Can you work these out from the model? Positions are in its coordinate system, mm. A direction names the side the tool comes from. Round coordinates to 2 decimals unless told otherwise and drop trailing zeros. Order: outer loops, then holes, each group sorted by start corner. A loop starts at its lowest first (then second) coordinate and runs counter-clockwise, first axis right, second up. Notation, with made-up numbers: (-33, 60.5) -> (-16, 60.5) arc R32 cw to (-16, 87.5) -> close; hole circle Ø7 at (-1, 1). An arc over 180 degrees is marked (long way). One line per item, written item: value.
```python
from build123d import *

# Parameters (mm, degrees)
EXTRUDE_1_DEPTH     = 68
SKETCH_2_R          = 1.5
CUT_EXTRUDE_1_DEPTH = 60
SKETCH_3_W          = 30
SKETCH_3_H          = 4
EXTRUDE_2_DEPTH     = 40
EXTRUDE_3_DEPTH     = 30
CUT_EXTRUDE_2_DEPTH = 4
EXTRUDE_4_DEPTH     = 23
EXTRUDE_START       = -53
EXTRUDE_5_DEPTH     = 23
EXTRUDE_6_DEPTH     = 3
EXTRUDE_7_DEPTH     = 0.66666
SKETCH_17_W         = 17.087989765
SKETCH_17_H         = 19.996406133
EXTRUDE_9_DEPTH     = 12
SKETCH_19_R         = 1.8
CUT_EXTRUDE_3_DEPTH = 20
SKETCH_20_W         = 61.603006609
SKETCH_20_H         = 84.586869481
CUT_EXTRUDE_4_DEPTH = 65
SKETCH_21_W         = 7.494214953
SKETCH_21_H         = 26.873102225
CUT_EXTRUDE_5_DEPTH = 2
SKETCH_22_W         = 9.970658679
SKETCH_22_H         = 25.794738871
CUT_EXTRUDE_6_DEPTH = 2
EXTRUDE_10_DEPTH    = 4
FILLET_1_R          = 1
FILLET_2_R          = 1


with BuildPart() as part:
    # 草图1 → 凸台-拉伸1 (new body)
    with BuildSketch(Plane(origin=(0, 0, 0), x_dir=(0, 0, -1), z_dir=(1, 0, 0))):
        Polygon((0, 0), (0, 4), (-10, 4), (-10, 7), (0, 7), (0, 10), (-14, 10), (-14, 0), align=None)
    extrude(amount=EXTRUDE_1_DEPTH)

    # 草图2 → 切除-拉伸1 (cut)
    with BuildSketch(Plane(origin=(0, 10, 0), x_dir=(1, 0, 0), z_dir=(0, 1, 0))):
        with Locations(Location((5, -3.5, 0), (0, 0, 270))):
            Circle(SKETCH_2_R)
        with Locations(Location((63, -3.5, 0), (0, 0, 270))):
            Circle(SKETCH_2_R)
    extrude(amount=-CUT_EXTRUDE_1_DEPTH, mode=Mode.SUBTRACT)

    # 草图3 → 凸台-拉伸2 (add)
    with BuildSketch(Plane.XZ):
        with Locations((34, 12)):
            Rectangle(SKETCH_3_W, SKETCH_3_H)
    extrude(amount=-EXTRUDE_2_DEPTH)

    # 草图4 → 凸台-拉伸3 (add)
    with BuildSketch(Plane(origin=(49, 0, 0), x_dir=(0, 0, -1), z_dir=(1, 0, 0))):
        Polygon((-14, 40), (-26.357684131, 54.727314459), (-23.293506358, 57.298464898), (-10, 41.455880937), (-10, 40), align=None)
    extrude(amount=-EXTRUDE_3_DEPTH)

    # 草图5 → 切除-拉伸2 (cut)
    with BuildSketch(Plane(origin=(0, 9.633382176, -11.480617817), x_dir=(1, 0, 0), z_dir=(0, -0.6427876096865429, 0.7660444431189751))):
        with BuildLine():
            Line((25.25, 55.318123989), (25.25, 43.864814933))
            ThreePointArc((25.25, 43.864814933), (23.75, 42.364814933), (22.25, 43.864814933))
            Line((22.25, 43.864814933), (22.25, 55.318123989))
            ThreePointArc((22.25, 55.318123989), (23.75, 56.818123989), (25.25, 55.318123989))
        make_face()
        with BuildLine():
            Line((42.75, 55.318123989), (42.75, 43.864814933))
            ThreePointArc((42.75, 43.864814933), (44.25, 42.364814933), (45.75, 43.864814933))
            Line((45.75, 43.864814933), (45.75, 55.318123989))
            ThreePointArc((45.75, 55.318123989), (44.25, 56.818123989), (42.75, 55.318123989))
        make_face()
    extrude(amount=-CUT_EXTRUDE_2_DEPTH, mode=Mode.SUBTRACT)

    # 草图6 → 凸台-拉伸4 (add)
    with BuildSketch(Plane.ZY.offset(-19)):
        Polygon((23.293506358, 57.298464898), (26.357684131, 54.727314459), (14, 40), (10.935822228, 42.571150439), align=None)
    extrude(amount=EXTRUDE_4_DEPTH)

    # 草图7 → 凸台-拉伸5 (add)
    with BuildSketch(Plane.ZY.offset(4).offset(EXTRUDE_START)):
        Polygon((23.293506358, 57.298464898), (26.357684131, 54.727314459), (14, 40), (10.935822228, 42.571150439), align=None)
    extrude(amount=-EXTRUDE_5_DEPTH)

    # 草图10 → 凸台-拉伸6 (add)
    with BuildSketch(Plane(origin=(52, 0, 0), x_dir=(0, 0.7660444431189749, 0.6427876096865431), z_dir=(-1, 0, 0))):
        Polygon((39.64080426, 18.986882184), (58.865947907, 18.986882184), (58.865947907, 25.653542184), (39.64080426, 20.653542184), align=None)
    extrude(amount=-EXTRUDE_6_DEPTH)

    # 草图15 → 凸台-拉伸7 (add)
    with BuildSketch(Plane(origin=(-0.224740323, 0.898508111, -2.01476807), x_dir=(0.9948507831271028, 0.04127952147527669, -0.09256306184522162), z_dir=(0.10135047760810084, -0.4051975406133526, 0.9085939873064868))):
        Polygon((55.510576319, 63.468125115), (55.510576319, 62.353864223), (55.510576319, 43.471718982), (72.598566084, 43.471718982), (72.598566084, 62.353864223), (72.598566084, 63.468125115), align=None)
    extrude(amount=-EXTRUDE_7_DEPTH)

    # 草图17 → 凸台-拉伸9 (add)
    with BuildSketch(Plane(origin=(-0.224740323, 0.898508111, -2.01476807), x_dir=(0.994850783127103, 0.04127952147527699, -0.09256306184522194), z_dir=(0.10135047760810126, -0.40519754061335256, 0.9085939873064869))):
        with Locations((64.054571201, 53.469922049)):
            Rectangle(SKETCH_17_W, SKETCH_17_H)
    extrude(amount=EXTRUDE_9_DEPTH)

    # 草图19 → 切除-拉伸3 (cut)
    with BuildSketch(Plane(origin=(-0.292306632, 1.168637103, -2.620491338), x_dir=(-0.9948507831271028, -0.04127952147527692, 0.09256306184522202), z_dir=(-0.10135047760810131, 0.40519754061335245, -0.908593987306487))):
        with Locations(Location((-62.598566084, 60.969922048, 0), (0, 0, 90))):
            Circle(SKETCH_19_R)
        with Locations(Location((-62.598566084, 45.969922048, 0), (0, 0, 270))):
            Circle(SKETCH_19_R)
    extrude(amount=-CUT_EXTRUDE_3_DEPTH, mode=Mode.SUBTRACT)

    # 草图20 → 切除-拉伸4 (cut)
    with BuildSketch(Plane.ZY.offset(-34)):
        with Locations((16.944749698, 32.191708304)):
            Rectangle(SKETCH_20_W, SKETCH_20_H)
    extrude(amount=CUT_EXTRUDE_4_DEPTH, mode=Mode.SUBTRACT)

    # 镜向7: part across plane


with BuildPart() as part_1:
    add(part.part)
    add(part.part.mirror(Plane.ZY.offset(-34)))

    # 草图21 → 切除-拉伸5 (cut)
    with BuildSketch(Plane(origin=(-0.292306632, 1.168637103, -2.620491338), x_dir=(-0.9948507831271028, -0.04127952147527692, 0.09256306184522202), z_dir=(-0.10135047760810131, 0.40519754061335245, -0.908593987306487))):
        with Locations((-54.514442647, 53.802326892)):
            Rectangle(SKETCH_21_W, SKETCH_21_H)
    extrude(amount=CUT_EXTRUDE_5_DEPTH, mode=Mode.SUBTRACT)

    # 草图22 → 切除-拉伸6 (cut)
    with BuildSketch(Plane(origin=(0.990797146, 3.961190673, -8.882368888), x_dir=(-0.9948507831271028, 0.04127952147527693, -0.09256306184522203), z_dir=(0.10135047760810131, 0.40519754061335256, -0.9085939873064868))):
        with Locations((-12.026553315, 54.032339334)):
            Rectangle(SKETCH_22_W, SKETCH_22_H)
    extrude(amount=CUT_EXTRUDE_6_DEPTH, mode=Mode.SUBTRACT)

    # 草图24 → 凸台-拉伸10 (add)
    with BuildSketch(Plane.XY.offset(14)):
        Polygon((19, 40), (3.059166743, 10), (8.395226669, 10), (19, 10), (19, 29.957752195), align=None)
        Polygon((49, 29.957752195), (49, 10), (59.604773331, 10), (64.940833257, 10), (49, 40), align=None)
    extrude(amount=-EXTRUDE_10_DEPTH)

    # 圆角1
    fillet_1_edges = [part_1.edges().sort_by_distance(p)[0] for p in [
        (34, 10, 10),
    ]]
    fillet(fillet_1_edges, radius=FILLET_1_R)

    # 圆角2
    fillet_2_edges = [part_1.edges().sort_by_distance(p)[0] for p in [
        (34, 41.455880937, 10),
    ]]
    fillet(fillet_2_edges, radius=FILLET_2_R)


solid = part_1.part
```
Q1. I want a section at A-A on z = 3.5. List the corners of the cut face in (x, y) for me, plus the area to 3 significant figures.
Answers below:
outline: (0, 0) -> (3.5, 0) -> (3.5, 4) -> (0, 4) -> close; (0, 7) -> (3.5, 7) -> (3.5, 10) -> (0, 10) -> close; (6.5, 0) -> (61.5, 0) -> (61.5, 4) -> (6.5, 4) -> close; (6.5, 7) -> (61.5, 7) -> (61.5, 10) -> (6.5, 10) -> close; (64.5, 0) -> (68, 0) -> (68, 4) -> (64.5, 4) -> close; (64.5, 7) -> (68, 7) -> (68, 10) -> (64.5, 10) -> close
area: 434 mm^2
Q2. I want a section at B-B on x = 31.5. List the corners of the cut face in (y, z) for me.
Answers below:
outline: (0, 0) -> (4, 0) -> (4, 10) -> (7, 10) -> (7, 0) -> (10, 0) -> (10, 9) arc R1 cw to (11, 10) -> (41.09, 10) arc R1 ccw to (41.73, 10.23) -> (57.3, 23.29) -> (54.73, 26.36) -> (40, 14) -> (0, 14) -> close
Q3. On a 3-axis mill with a long thin cutter (end or side, diameter ignored), from which of +Z, -Z, +X, -X, +Y, -Y can I reach the whole of each face in a straight line? I mean faces 1 (the face through (44.217, 43.355, 14.241)), 2 (the face through (25.25, 49, 19)), 3 (the face through (0, 3, 7)), 4 (the face through (34, 4, 5)). Say none if no direction works.
Answers below:
face 1: +Z, +Y
face 2: none
face 3: +Z, -Z, -X, -Y
face 4: -Z, +X, -X
Q4. We'd pull the mould along X, two halves only. Please class faces 5 (the face through (52, 53, 16)), 6 (the face through (34, 16, 14)), 7 (the face through (72.565, 50.341, 18.054)), 8 (the face through (-4, 41.1, 13.2)): released by +X, released by -X, zero draft, split by the parting line, or undercut.
Answers below:
face 5: undercut
face 6: zero draft
face 7: released by +X
face 8: released by -X
Q5. Will these pins go through, and if not, where does the flat tip stop? pin 1 Ø1 at (x, z) = (54, 18) entering from +Y; pin 2 Ø3 at (y, z) = (55.5, 19) entering from -X; pin 3 Ø10 at (y, z) = (51.5, 18.5) entering from +X.
Answers below:
pin 1: y = 61.57
pin 2: x = -4.59
pin 3: x = 73.07
Q6. I want a section at C-C on y = 9. List the corners of the cut face in (x, z) for me.
Answers below:
outline: (0, 0) -> (68, 0) -> (68, 14) -> (0, 14) -> close; hole circle Ø3 at (5, 3.5); hole circle Ø3 at (63, 3.5)
Q7. I want a section at D-D on y = 28. List the corners of the cut face in (x, z) for me.
Answers below:
outline: (12.62, 10) -> (55.38, 10) -> (55.38, 14) -> (12.62, 14) -> close
Q8. Please list where these lines run through material, in increasing order: line 1 along X through (y, z) = (9.35, 3.5); line 2 along Y through (x, z) = (58, 7.75); line 3 along Z through (x, y) = (5, 0.8).
Answers below:
line 1: 0 to 3.5, 6.5 to 61.5, 64.5 to 68
line 2: 0 to 4, 7 to 10
line 3: 0 to 2, 5 to 14
